Verification items for the finished model (mm, model axes). Face numbers are marked on the shaded views. A direction names the side the tool comes from. Coordinates: 2 decimals unless noted, no trailing zeros. Order: outer loops, then holes, each group sorted by start corner. A loop starts at its lowest first (then second) coordinate and runs counter-clockwise, first axis right, second up. Notation, with made-up numbers: M 81,75.25 L 115,75.25 A20 ccw 115,111.25 Z; hole C -32.5,73.5 d2. An arc over 180 degrees is marked long. Return JSON: item names as keys, results as strings. Group by question number.
Q1. Mould release check, pull along Z, two halves, no side actions. Record for the marked faces 4, 5, 6 and 7: pulls with the +Z half, pulls with the -Z half, needs draft (parallel to the pull), parting line crosses it, or undercut.
Q2. Access from +Z, -Z, +X, -X, +Y, -Y to the whole of each face (thin tool, end or side, straight path). Record for the marked faces 1, 2 and 3.
Q3. Section check D-D, the plane z = -27. Enter the section's corners in (x, y) (1 decimal).
Q4. Section check C-C, the plane z = 5. Enter the section's corners in (x, y), then the cut area to 3 significant figures.
Q5. Thickness scan on probe 1 along X at (y, z) = (0.75, -28) (3 decimals); probe 2 along X at (y, z) = (-3.5, -10); probe 3 along Z at (x, y) = (0, -2.75) (3 decimals). Record the ranges inside material, lowest first.
Q6. Go/stop test with flat-tipped pins: pin 1 Ø2.5 at (x, y) = (-23.81, 0) entering from +Z; pin 2 Ø5 at (x, y) = (-23.5, -0.5) entering from +Z; pin 3 Ø3 at (y, z) = (1.5, -11) entering from -X; pin 4 Ø1 at (y, z) = (-1, -9) entering from +X. Record where each tip stops, or that it passes through.
Q7. Section check A-A, the plane y = 3.5. Enter the section's corners in (x, z) (3 decimals).
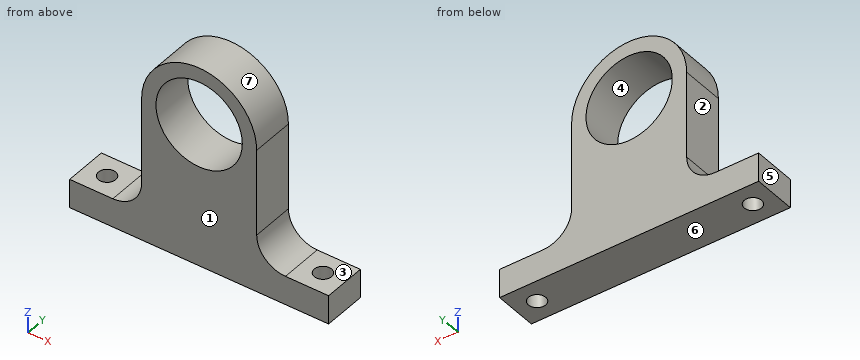
from build123d import *

# Parameters (mm, degrees)
F1_DEPTH = 4.7625
F2_R     = 6.35
F4_D     = 3.81


with BuildPart() as f1:
    # F0 (on Front) → F1 (new body, symmetric)
    with BuildSketch(Plane.XZ):
        with BuildLine():
            Line((12.7, -25.4), (12.7, 0))
            ThreePointArc((12.7, 0), (0, 12.7), (-12.7, 0))
            Line((-12.7, 0), (-12.7, -25.4))
            Line((-12.7, -25.4), (-28.575, -25.4))
            Line((-28.575, -25.4), (-28.575, -31.75))
            Line((-28.575, -31.75), (28.575, -31.75))
            Line((28.575, -31.75), (28.575, -25.4))
            Line((28.575, -25.4), (12.7, -25.4))
        make_face()
        with BuildLine():
            ThreePointArc((-9.525, 1e-08), (5e-09, 9.525), (9.525, 0))
            ThreePointArc((9.525, 0), (-5e-09, -9.525), (-9.525, 1e-08))
        make_face(mode=Mode.SUBTRACT)
    extrude(amount=F1_DEPTH, both=True)

    # F2
    f2_edges = [f1.edges().sort_by_distance(p)[0] for p in [
        (-12.7, 0, -25.4),
        (12.7, 0, -25.4),
    ]]
    fillet(f2_edges, radius=F2_R)

    # F4 (through all)
    with Locations(Plane(origin=(0, 0, -31.75), x_dir=(1, 0, 0), z_dir=(0, 0, -1))):
        with Locations((-23.8125, 0), (23.8125, 0)):
            Hole(F4_D / 2)


solid = f1.part
Numbers:
{
 "1": {"face 4": "undercut", "face 5": "needs draft", "face 6": "pulls with the -Z half", "face 7": "pulls with the +Z half"},
 "2": {"face 1": "+Z, -Z, +X, -X, -Y", "face 2": "+Z, -X, +Y, -Y", "face 3": "+Z, +X, +Y, -Y"},
 "3": {"outline": "M -28.6,-4.8 L 28.6,-4.8 L 28.6,4.8 L -28.6,4.8 Z; hole C -23.8,0 d3.8; hole C 23.8,0 d3.8"},
 "4": {"outline": "M -11.67,-4.76 L -8.11,-4.76 L -8.11,4.76 L -11.67,4.76 Z; M 8.11,-4.76 L 11.67,-4.76 L 11.67,4.76 L 8.11,4.76 Z", "area": "68.0 mm2"},
 "5": {"probe 1": "x = -28.575 to -25.564, -22.061 to 22.061, 25.564 to 28.575", "probe 2": "x = -12.7 to 12.7", "probe 3": "z = -31.75 to -9.525, 9.525 to 12.7"},
 "6": {"pin 1": "passes through", "pin 2": "stops at z = -25.4", "pin 3": "stops at x = -12.7", "pin 4": "stops at x = 12.7"},
 "7": {"outline": "M -28.575,-31.75 L 28.575,-31.75 L 28.575,-25.4 L 19.05,-25.4 A6.35 cw 12.7,-19.05 L 12.7,0 A12.7 ccw -12.7,0 L -12.7,-19.05 A6.35 cw -19.05,-25.4 L -28.575,-25.4 Z; hole C 0,0 d19.05"}
}
